from build123d import *

# Parameters (mm, degrees)
F0_W     = 155
F0_H     = 5
F1_DEPTH = 28
F0_H_2   = 150
F2_DEPTH = 3
F3_R     = 1.5
F4_R     = 1.5


with BuildPart() as f1:
    # F0 (on Top) → F1 (new body)
    with BuildSketch(Plane.XY):
        with Locations((77.5, 2.5)):
            Rectangle(F0_W, F0_H)
    extrude(amount=F1_DEPTH)

    # F0 (on Top) → F2 (join)
    with BuildSketch(Plane.XY):
        with Locations((77.5, 2.5)):
            Rectangle(F0_W, F0_H)
        with Locations((77.5, 80)):
            Rectangle(F0_W, F0_H_2)
    extrude(amount=F2_DEPTH)

    # F3
    f3_edges = [f1.edges().sort_by_distance(p)[0] for p in [
        (77.5, 0, 28),
    ]]
    fillet(f3_edges, radius=F3_R)

    # F4
    f4_edges = [f1.edges().sort_by_distance(p)[0] for p in [
        (0, 0, 13.25),
        (155, 0, 13.25),
    ]]
    fillet(f4_edges, radius=F4_R)


solid = f1.part
For this review, take the finished solid that the model builds, in its own axes (mm). A direction names the side the tool comes from. Round coordinates to 2 decimals unless told otherwise and drop trailing zeros. Write each loop counter-clockwise with the first axis right and the second up, starting at its lowest first coordinate (ties: lowest second). Pieces come first, ordered by that corner, then holes. Notation, with made-up numbers: (59.5, 30.5) - (69.5, 30.5) arc R28 ccw to (69.5, 51.5) - close; hole circle Ø9 at (7.25, -14). An arc over 180 degrees is marked (long way). Write item = value, one per line. Start each with the question number.
1. For faces 1 (the face through (155, 61, 2)), 2 (the face through (76, 5, 15)), list the 3-axis set-ups (+Z, -Z, +X, -X, +Y, -Y) from which the entire face can be reached by the end or side of a thin tool; tool diameter is ignored.
2. Consider section A-A on z = 16.25. State the section outline as (x, y) points, plus the area to 3 significant figures.
3. For pin 1 Ø2 at (x, z) = (73.5, 9.5) entering from +Y, flat-tipped, find the tip position at first contact; note if it passes through.
4. Consider section B-B on x = 61. State the section outline as (y, z) points, plus the area to 3 significant figures.
5. Consider section C-C on y = 92. State the section outline as (x, z) points.
6. Wall thickness on L1, parallel to Y at x = 85.5, z = 4.75; L2, parallel to Z at x = 64.5, y = 96: over which ranges is each line inside the solid? List them lowest first.
Evaluation:
q1.face_1 = +Z, -Z, +X, +Y, -Y
q1.face_2 = +Z, +X, -X, +Y
q2.outline = (0, 1.5) arc R1.5 ccw to (1.5, 0) - (153.5, 0) arc R1.5 ccw to (155, 1.5) - (155, 5) - (0, 5) - close
q2.area = 774 mm2
q3.pin_1 = 5
q4.outline = (0, 0) - (155, 0) - (155, 3) - (5, 3) - (5, 28) - (1.5, 28) arc R1.5 ccw to (0, 26.5) - close
q4.area = 590 mm2
q5.outline = (0, 0) - (155, 0) - (155, 3) - (0, 3) - close
q6.L1 = 0 to 5
q6.L2 = 0 to 3
